Check sheet for the drawn part. Datum: minimum x, y, z corner. Units: mm. Give positions to 0.01 mm unless a question says otherwise; leave off trailing zeros. Order: outer loops, then holes, each group sorted by start corner. A loop starts at its lowest first (then second) coordinate and runs counter-clockwise, first axis right, second up. Notation, with made-up numbers: (32.5, -38) - (56.5, -38) arc R19 cw to (56.5, -6) - close; hole circle Ø9 at (80, -5.75). An arc over 180 degrees is marked (long way). Answer as a JSON object with one key per item and string values. Group by question number.
(1) Section check B-B (z = 1.25). Record the boundary of the cut face in (x, y), then the cut area to 3 significant figures.
(2) Section check A-A (y = 69). Record the boundary of the cut face in (x, z), then the cut area to 3 significant figures.
(3) Depth check by flat-ended pin: pin 1 Ø1.5 at (x, z) = (55.5, 2) entering from +Y; pin 2 Ø1 at (y, z) = (18.5, 1.5) entering from -X. Enter the tip coordinate at first touch or a pass-through.
(4) Section check C-C (x = 71.5). Record the boundary of the cut face in (y, z), then the cut area to 3 significant figures.
(5) Thickness scan on line 1 (X direction, y = 57.5, z = 0.75); line 2 (Y direction, x = 31.5, z = 2.45); line 3 (X direction, y = 13, z = 2.5). Record the ranges inside material, lowest first.
(6) Section check D-D (x = 15). Record the boundary of the cut face in (y, z), then the cut area to 3 significant figures.
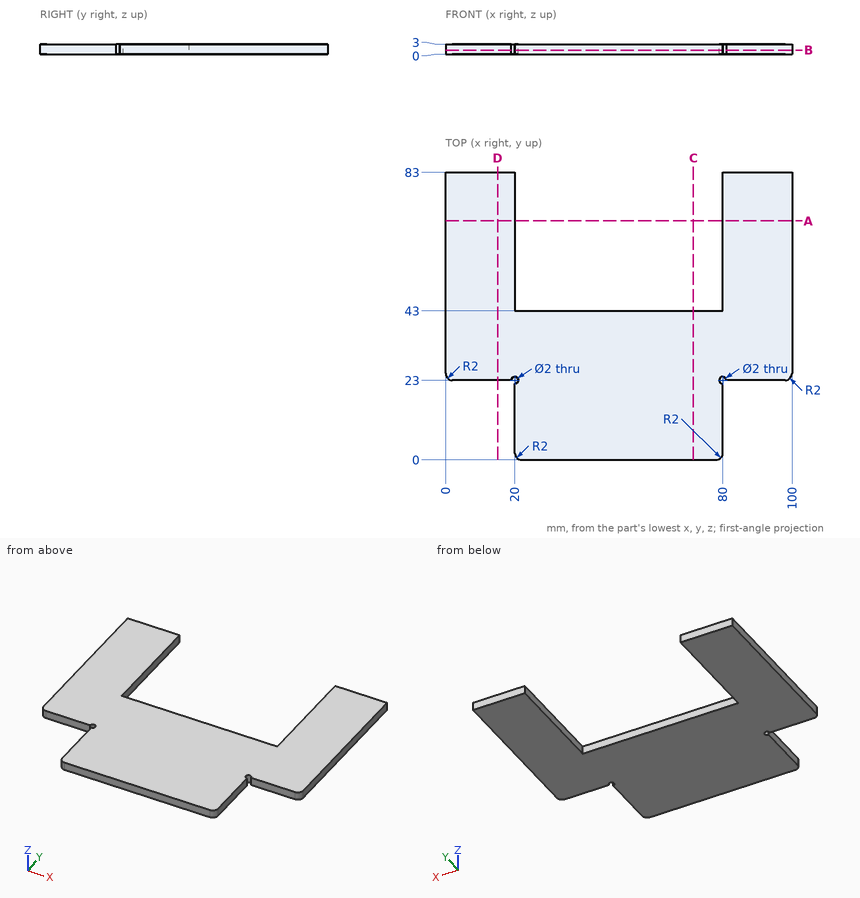
Solutions:
{
 "1": {"outline": "(0, 25) arc R2 ccw to (2, 23) - (19, 23) arc R1 cw (long way) to (20, 22) - (20, 2) arc R2 ccw to (22, 0) - (78, 0) arc R2 ccw to (80, 2) - (80, 22) arc R1 cw (long way) to (81, 23) - (98, 23) arc R2 ccw to (100, 25) - (100, 83) - (80, 83) - (80, 43) - (20, 43) - (20, 83) - (0, 83) - close", "area": "4,970 mm2"},
 "2": {"outline": "(0, 0) - (20, 0) - (20, 3) - (0, 3) - close; (80, 0) - (100, 0) - (100, 3) - (80, 3) - close", "area": "120 mm2"},
 "3": {"pin 1": "stops at y = 43", "pin 2": "stops at x = 20"},
 "4": {"outline": "(0, 0) - (43, 0) - (43, 3) - (0, 3) - close", "area": "129 mm2"},
 "5": {"line 1": "x = 0 to 20, 80 to 100", "line 2": "y = 0 to 43", "line 3": "x = 20 to 80"},
 "6": {"outline": "(23, 0) - (83, 0) - (83, 3) - (23, 3) - close", "area": "180 mm2"}
}
